Check sheet for the modelled part. Datum: model origin and axes. Units: mm. A direction names the side the tool comes from. Round coordinates to 2 decimals unless told otherwise and drop trailing zeros. Loops run counter-clockwise (first coordinate to the right, second up) from the corner with the lowest first, then second, coordinate; pieces in that order, holes last. Notation, with made-up numbers: (78, 51) - (99, 51) arc R19 ccw to (99, 70) - close; hole circle Ø4 at (77, 76). An arc over 180 degrees is marked (long way). Answer in a Markdown table with one row per item. Add a question column.
(1) Access from +Z, -Z, +X, -X, +Y, -Y to the whole of each face (thin tool, end or side, straight path). Record for faces 1 (the flat face through (25, 16.542, 1)), 2 (the flat face through (-25.993, 18, 2)), 3 (the flat face through (-39, -14.058, 1)), 4 (the flat face through (-39, -29.058, 1)), 5 (the flat face through (-12, 16.542, 1)).
(2) Cross-section at C-C on y = 14. Enter the section's corners in (x, z), then the cut area to 3 significant figures.
(3) Thickness scan on line 1 along Y through (x, z) = (24.5, 2.5); line 2 along X through (y, z) = (14, 1.2). Record the ranges inside material, lowest first.
(4) Gauge pin test, flat ends, axial feed: pin 1 (0.9 mm diameter, centred on x = 30.5, z = 2, fed in from -Y); pin 2 (0.9 mm diameter, centred on x = 31, z = 1.5, fed in from +Y); pin 3 (0.9 mm diameter, centred on y = 18.5, z = 1.5, fed in from +X). Record the tip position at first contact, or that the pin passes through.
(5) Cross-section at B-B on x = -14.5. Enter the section's corners in (y, z), then the cut area to 3 significant figures.
(6) Mould release check, pull along Y, two halves, no side actions. Record for faces 6 (the flat face through (-22, 19.542, 1)), 7 (the flat face through (14.007, 18, 2)), 8 (the flat face through (-40, -6.258, 2)), 9 (the flat face through (-37.993, -10, 2)): +Y half, -Y half, draft (parallel to the pull), parting line (faces both ways), or undercut.
from build123d import *

# Parameters (mm, degrees)
SKETCH1_W           = 73
SKETCH1_H           = 50
BOSS_EXTRUDE1_DEPTH = 3
SKETCH2_W           = 3
SKETCH2_H           = 7.8
CUT_EXTRUDE1_DEPTH  = 53.999062732
LPATTERN1_COUNT     = 3
LPATTERN1_PITCH     = 22.8
SKETCH3_W           = 3
SKETCH3_H           = 7.8
CUT_EXTRUDE2_DEPTH  = 53.999062732
LPATTERN2_COUNT     = 4
LPATTERN2_PITCH     = 22.8
SKETCH6_W           = 3
SKETCH6_H           = 19.4
CUT_EXTRUDE3_DEPTH  = 10
SKETCH7_W           = 7.8
SKETCH7_H           = 3
BOSS_EXTRUDE2_DEPTH = 3
LPATTERN3_COUNT     = 3
LPATTERN3_PITCH     = 20
SKETCH8_W           = 3
SKETCH8_H           = 15
BOSS_EXTRUDE3_DEPTH = 3


with BuildPart() as part:
    # Sketch1 → Boss-Extrude1 (new body)
    with BuildSketch(Plane.XY):
        with Locations((-4.493460648, -8.457986111)):
            Rectangle(SKETCH1_W, SKETCH1_H)
    extrude(amount=BOSS_EXTRUDE1_DEPTH)

    # Sketch2 → Cut-Extrude1 (cut, through all)
    with BuildSketch(Plane.XY.offset(3)):
        with Locations((-39.493460648, 12.642013889)):
            Rectangle(SKETCH2_W, SKETCH2_H)
    cut_extrude1 = extrude(amount=-CUT_EXTRUDE1_DEPTH, mode=Mode.SUBTRACT)

    # LPattern1: Cut-Extrude1 ×3
    with Locations(*[(0, -i * LPATTERN1_PITCH, 0) for i in range(1, LPATTERN1_COUNT)]):
        add(cut_extrude1, mode=Mode.SUBTRACT)

    # Sketch3 → Cut-Extrude2 (cut, through all)
    with BuildSketch(Plane.XY.offset(3)):
        with Locations((30.506539352, 12.642013889)):
            Rectangle(SKETCH3_W, SKETCH3_H)
    cut_extrude2 = extrude(amount=-CUT_EXTRUDE2_DEPTH, mode=Mode.SUBTRACT)

    # LPattern2: Cut-Extrude2 ×4
    with Locations(*[(0, -i * LPATTERN2_PITCH, 0) for i in range(1, LPATTERN2_COUNT)]):
        add(cut_extrude2, mode=Mode.SUBTRACT)

    # Sketch6 → Cut-Extrude3 (cut)
    with BuildSketch(Plane.XY.offset(3)):
        with Locations((-39.493460648, -23.757986111)):
            Rectangle(SKETCH6_W, SKETCH6_H)
    extrude(amount=-CUT_EXTRUDE3_DEPTH, mode=Mode.SUBTRACT)

    # Sketch7 → Boss-Extrude2 (add)
    with BuildSketch(Plane(origin=(0, 16.542013889, 0), x_dir=(1, 0, 0), z_dir=(0, 1, 0))):
        with Locations((-22.093460648, -1.5)):
            Rectangle(SKETCH7_W, SKETCH7_H)
    boss_extrude2 = extrude(amount=BOSS_EXTRUDE2_DEPTH)

    # LPattern3: Boss-Extrude2 ×3
    with Locations(*[(i * LPATTERN3_PITCH, 0, 0) for i in range(1, LPATTERN3_COUNT)]):
        add(boss_extrude2)

    # Sketch8 → Boss-Extrude3 (add)
    with BuildSketch(Plane.ZY.offset(37.993460648)):
        with Locations((1.5, -21.557986111)):
            Rectangle(SKETCH8_W, SKETCH8_H)
    extrude(amount=BOSS_EXTRUDE3_DEPTH)


solid = part.part
Answers:
| question | item | result |
|---|---|---|
| 1 | face 1 | +Z, -Z, +X, +Y |
| 1 | face 2 | +Z, -Z, -X, +Y |
| 1 | face 3 | +Z, -Z, -X |
| 1 | face 4 | +Z, -Z, -X, -Y |
| 1 | face 5 | +Z, -Z, +Y |
| 2 | outline | (-37.99, 0) - (29.01, 0) - (29.01, 3) - (-37.99, 3) - close |
| 2 | area | 201 mm^2 |
| 3 | line 1 | y = -33.46 to 16.54 |
| 3 | line 2 | x = -37.99 to 29.01 |
| 4 | pin 1 | stops at y = -29.06 |
| 4 | pin 2 | stops at y = 8.74 |
| 4 | pin 3 | stops at x = 21.81 |
| 5 | outline | (-33.46, 0) - (16.54, 0) - (16.54, 3) - (-33.46, 3) - close |
| 5 | area | 150 mm^2 |
| 6 | face 6 | +Y half |
| 6 | face 7 | draft |
| 6 | face 8 | undercut |
| 6 | face 9 | undercut |
